from build123d import *

# Parameters (mm, degrees)
F0_R     = 10
F1_DEPTH = 12.5
F2_R     = 2.5
F3_DEPTH = 12
F4_R     = 5
F5_DEPTH = 12


with BuildPart() as f1:
    # F0 (on Front) → F1 (new body, symmetric)
    with BuildSketch(Plane.XZ):
        Circle(F0_R)
    extrude(amount=F1_DEPTH, both=True)

    # F2 (on face) → F3 (cut)
    with BuildSketch(Plane.XZ.offset(12.5)):
        Circle(F2_R)
    extrude(amount=-F3_DEPTH, mode=Mode.SUBTRACT)

    # F4 (on face) → F5 (cut)
    with BuildSketch(Plane(origin=(0, 12.5, 0), x_dir=(-1, 0, 0), z_dir=(0, 1, 0))):
        Circle(F4_R)
    extrude(amount=-F5_DEPTH, mode=Mode.SUBTRACT)


solid = f1.part
Can you work these out from the model? Positions are in its coordinate system, mm. A direction names the side the tool comes from. Coordinates: 2 decimals unless noted, no trailing zeros. Write each loop counter-clockwise with the first axis right and the second up, starting at its lowest first coordinate (ties: lowest second). Pieces come first, ordered by that corner, then holes. Notation, with made-up numbers: M 72.25,-6.75 L 96.25,-6.75 A22 ccw 96.25,16.25 Z; hole C -29,45.5 d9. An arc over 180 degrees is marked long. Use one line per item in the form item = value.
Q1. For faces 1 (the cylindrical face through (-0.54, -6.58, -2.44)), 2 (the flat face through (0, 0.5, 0)), 3 (the flat face through (-5, 12.5, -2)), which set-ups out of +Z, -Z, +X, -X, +Y, -Y let a thin tool reach every point of the face, with its end or its side?
Model answer:
face_1 = -Y
face_2 = +Y
face_3 = +Z, -Z, +X, -X, +Y
Q2. For P1, Ø3, axis at x = -2.5, z = -0.5, coming from the +Y side; P2, Ø5, axis at y = 8.5, z = -3, coming from the -X side; P3, Ø1, axis at x = -1.5, y = -7.5, coming from the +Z side, each with a flat end and sliding along its axis, tell me the tip position at first contact or that it passes through.
Model answer:
P1 = 0.5
P2 = -9.99
P3 = 9.95
Q3. I need wall thicknesses on line 1 along Z through (x, y) = (0, 4.5); line 2 along Z through (x, y) = (0, -4.5); line 3 along Y through (x, z) = (-2, 4.25). Which ranges of each line are inside material? Lowest first, please. Write a range as from..to.
Model answer:
line_1 = -10..-5, 5..10
line_2 = -10..-2.5, 2.5..10
line_3 = -12.5..0.5
Q4. If we section it at B-B (y = 8): Write out the boundary of the cut face in (x, z).
Model answer:
outline = C 0,0 d20; hole C 0,0 d10
Q5. We'd pull the mould along Z, two halves only. Please class faces 4 (the flat face through (2, -12.5, -2)), 5 (the flat face through (0, -0.5, 0)), 6 (the cylindrical face through (-2.17, -0.18, -9.76)): +Z half, -Z half, draft (parallel to the pull), parting line (faces both ways), or undercut.
Model answer:
face_4 = draft
face_5 = undercut
face_6 = parting line
Q6. If we section it at C-C (x = 0): Write out the boundary of the cut face in (y, z), then the cut area to 3 significant figures.
Model answer:
outline = M -12.5,-10 L 12.5,-10 L 12.5,-5 L 0.5,-5 L 0.5,5 L 12.5,5 L 12.5,10 L -12.5,10 L -12.5,2.5 L -0.5,2.5 L -0.5,-2.5 L -12.5,-2.5 Z
area = 320 mm^2
Q7. If we section it at D-D (y = -3.5): Write out the boundary of the cut face in (x, z), then the cut area to 3 significant figures.
Model answer:
outline = C 0,0 d20; hole C 0,0 d5
area = 295 mm^2
Q8. If we section it at A-A (z = 0): Write out the boundary of the cut face in (x, y).
Model answer:
outline = M -10,-12.5 L -2.5,-12.5 L -2.5,-0.5 L 2.5,-0.5 L 2.5,-12.5 L 10,-12.5 L 10,12.5 L 5,12.5 L 5,0.5 L -5,0.5 L -5,12.5 L -10,12.5 Z
